Check sheet for the modelled part. Datum: model origin and axes. Units: mm. Round coordinates to 2 decimals unless told otherwise and drop trailing zeros. Write each loop counter-clockwise with the first axis right and the second up, starting at its lowest first coordinate (ties: lowest second). Pieces come first, ordered by that corner, then holes.
Item 1: Cross-section at A-A on y = 115. Enter the section's corners in (x, z).
Item 2: Cross-section at B-B on z = 0. Enter the section's corners in (x, y).
Item 3: Go/stop test with flat-tipped pins: pin 1 Ø1 at (y, z) = (124.5, -4.5) entering from -X; pin 2 Ø3.5 at (y, z) = (-90, -0.5) entering from +X; pin 3 Ø12 at (x, y) = (-3.5, -55) entering from -Z; pin 4 Ø6 at (x, y) = (0, 151.5) entering from -Z. Record where each tip stops, or that it passes through.
Item 4: Cross-section at C-C on x = 0. Enter the section's corners in (y, z).
Item 5: Material ranges on line 1 (Z direction, x = 11.5, y = 207); line 2 (Z direction, x = -1.25, y = 189.5), recorded low to high.
from build123d import *

# Parameters (mm, degrees)
SKETCH1_W           = 25.4
SKETCH1_H           = 25.4
BOSS_EXTRUDE1_DEPTH = 500
CUT_EXTRUDE2_DEPTH  = 2
CUT_EXTRUDE3_DEPTH  = 2
CUT_EXTRUDE4_START  = -2
CUT_EXTRUDE4_DEPTH  = 2
CUT_EXTRUDE5_START  = -2
CUT_EXTRUDE5_DEPTH  = 2


with BuildPart() as part:
    # Sketch1 → Boss-Extrude1 (new, symmetric)
    with BuildSketch(Plane(origin=(0, 0, 0), x_dir=(1, 0, 0), z_dir=(0, 1, 0))):
        Rectangle(SKETCH1_W, SKETCH1_H)
    extrude(amount=BOSS_EXTRUDE1_DEPTH, both=True)

    # Sketch5 → Cut-Extrude2 (cut)
    with BuildSketch(Plane.XY.offset(12.7)):
        with BuildLine():
            Line((6, 450), (6, -450))
            ThreePointArc((6, -450), (0, -456), (-6, -450))
            Line((-6, -450), (-6, 450))
            ThreePointArc((-6, 450), (0, 456), (6, 450))
        make_face()
    extrude(amount=-CUT_EXTRUDE2_DEPTH, mode=Mode.SUBTRACT)

    # Sketch6 → Cut-Extrude3 (cut)
    with BuildSketch(Plane(origin=(12.7, 0, 0), x_dir=(0, 0, -1), z_dir=(1, 0, 0))):
        with BuildLine():
            Line((6, 450), (6, -450))
            ThreePointArc((6, -450), (0, -456), (-6, -450))
            Line((-6, -450), (-6, 450))
            ThreePointArc((-6, 450), (0, 456), (6, 450))
        make_face()
    extrude(amount=-CUT_EXTRUDE3_DEPTH, mode=Mode.SUBTRACT)

    # Sketch8 → Cut-Extrude4 (cut)
    with BuildSketch(Plane(origin=(0, 0, -12.7), x_dir=(-1, 0, 0), z_dir=(0, 0, -1)).offset(CUT_EXTRUDE4_START)):
        with BuildLine():
            Line((6, 450), (6, -450))
            ThreePointArc((6, -450), (0, -456), (-6, -450))
            Line((-6, -450), (-6, 450))
            ThreePointArc((-6, 450), (0, 456), (6, 450))
        make_face()
    extrude(amount=CUT_EXTRUDE4_DEPTH, mode=Mode.SUBTRACT)

    # Sketch9 → Cut-Extrude5 (cut)
    with BuildSketch(Plane.ZY.offset(12.7).offset(CUT_EXTRUDE5_START)):
        with BuildLine():
            Line((6, 450), (6, -450))
            ThreePointArc((6, -450), (0, -456), (-6, -450))
            Line((-6, -450), (-6, 450))
            ThreePointArc((-6, 450), (0, 456), (6, 450))
        make_face()
    extrude(amount=CUT_EXTRUDE5_DEPTH, mode=Mode.SUBTRACT)


solid = part.part
Response values:
1. outline: (-12.7, -12.7) - (-6, -12.7) - (-6, -10.7) - (6, -10.7) - (6, -12.7) - (12.7, -12.7) - (12.7, -6) - (10.7, -6) - (10.7, 6) - (12.7, 6) - (12.7, 12.7) - (6, 12.7) - (6, 10.7) - (-6, 10.7) - (-6, 12.7) - (-12.7, 12.7) - (-12.7, 6) - (-10.7, 6) - (-10.7, -6) - (-12.7, -6) - close
2. outline: (-12.7, -500) - (12.7, -500) - (12.7, -456) - (10.7, -456) - (10.7, 456) - (12.7, 456) - (12.7, 500) - (-12.7, 500) - (-12.7, 456) - (-10.7, 456) - (-10.7, -456) - (-12.7, -456) - close
3. pin 1: stops at x = -10.7
3. pin 2: stops at x = 10.7
3. pin 3: stops at z = -12.7
3. pin 4: stops at z = -10.7
4. outline: (-500, -12.7) - (-456, -12.7) - (-456, -10.7) - (456, -10.7) - (456, -12.7) - (500, -12.7) - (500, 12.7) - (456, 12.7) - (456, 10.7) - (-456, 10.7) - (-456, 12.7) - (-500, 12.7) - close
5. line 1: z = -12.7 to -6, 6 to 12.7
5. line 2: z = -10.7 to 10.7
